Part model, mm, in its own coordinate system. Face numbers are marked on the shaded views. A direction names the side the tool comes from. Round coordinates to 2 decimals unless told otherwise and drop trailing zeros. Loops run counter-clockwise (first coordinate to the right, second up) from the corner with the lowest first, then second, coordinate; pieces in that order, holes last. Notation, with made-up numbers: M 21,89 L 72,89 A21 cw 72,96 Z; hole C 14.25,-20.5 d7. An arc over 180 degrees is marked long. Put each result on its own line as item: value. Start each with the question number.
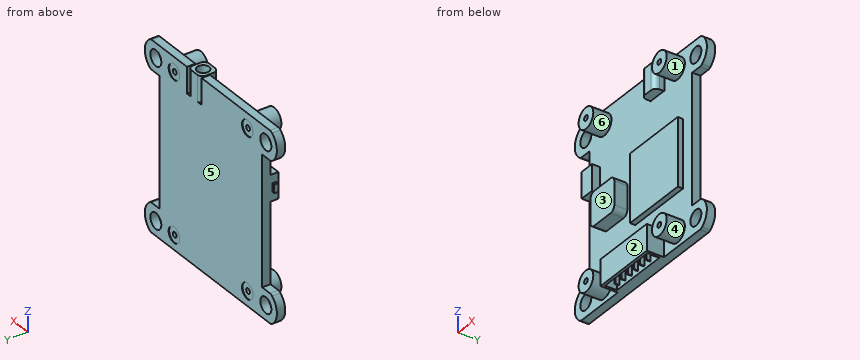
```python
from build123d import *

# Parameters (mm, degrees)
SKETCH1_R            = 1.5
SKETCH1_R_2          = 0.5
BOSS_EXTRUDE1_DEPTH  = 1.6
SKETCH2_R            = 2
SKETCH2_R_2          = 0.5
BOSS_EXTRUDE2_DEPTH  = 3.5
SKETCH3_R            = 1.5
SKETCH3_R_2          = 0.5
CUT_EXTRUDE1_DEPTH   = 0.1
SKETCH4_W            = 2.814940843
SKETCH4_H            = 5
BOSS_EXTRUDE3_DEPTH  = 1.5
SKETCH5_W            = 1.6
SKETCH5_H            = 0.8
BOSS_EXTRUDE4_DEPTH  = 0.5
BOSS_EXTRUDE5_DEPTH  = 2.5
SKETCH7_W            = 13
SKETCH7_H            = 13
BOSS_EXTRUDE6_DEPTH  = 1
SKETCH8_W            = 4
SKETCH8_H            = 1.6
CUT_EXTRUDE2_DEPTH   = 5
BOSS_EXTRUDE8_DEPTH  = 5
SKETCH10_R           = 1.15
CUT_EXTRUDE3_DEPTH   = 4
SKETCH11_W           = 12.6
SKETCH11_H           = 3.3
BOSS_EXTRUDE9_DEPTH  = 5
SKETCH12_W           = 11.6
SKETCH12_H           = 2.3
CUT_EXTRUDE4_DEPTH   = 4
SKETCH13_W           = 0.181198264
SKETCH13_H           = 0.795431403
BOSS_EXTRUDE10_DEPTH = 3.5


with BuildPart() as part:
    # Sketch1 → Boss-Extrude1 (new body)
    with BuildSketch(Plane(origin=(0, 0, 0), x_dir=(1, 0, 0), z_dir=(0, 1, 0))):
        with BuildLine():
            ThreePointArc((16.1, -18), (16.416227766, -17.948683298), (16.7, -17.8))
            ThreePointArc((16.7, -17.8), (18, -15.2), (16.7, -12.6))
            ThreePointArc((16.7, -12.6), (16.416227766, -12.451316702), (16.1, -12.4))
            Line((16.1, -12.4), (14, -12.4))
            Line((14, -12.4), (14, 12.4))
            Line((14, 12.4), (16.1, 12.4))
            ThreePointArc((16.1, 12.4), (16.416227766, 12.451316702), (16.7, 12.6))
            ThreePointArc((16.7, 12.6), (18, 15.2), (16.7, 17.8))
            ThreePointArc((16.7, 17.8), (16.416227766, 17.948683298), (16.1, 18))
            Line((16.1, 18), (-16.1, 18))
            ThreePointArc((-16.1, 18), (-16.416227766, 17.948683298), (-16.7, 17.8))
            ThreePointArc((-16.7, 17.8), (-18, 15.2), (-16.7, 12.6))
            ThreePointArc((-16.7, 12.6), (-16.416227766, 12.451316702), (-16.1, 12.4))
            Line((-16.1, 12.4), (-14, 12.4))
            Line((-14, 12.4), (-14, -12.4))
            Line((-14, -12.4), (-16.1, -12.4))
            ThreePointArc((-16.1, -12.4), (-16.416227766, -12.451316702), (-16.7, -12.6))
            ThreePointArc((-16.7, -12.6), (-18, -15.2), (-16.7, -17.8))
            ThreePointArc((-16.7, -17.8), (-16.416227766, -17.948683298), (-16.1, -18))
            Line((-16.1, -18), (16.1, -18))
        make_face()
        with Locations(Location((-15, 15.2, 0), (0, 0, 270))):
            Circle(SKETCH1_R, mode=Mode.SUBTRACT)
        with Locations(Location((15, 15.2, 0), (0, 0, 270))):
            Circle(SKETCH1_R, mode=Mode.SUBTRACT)
        with Locations(Location((-15, -15.2, 0), (0, 0, 270))):
            Circle(SKETCH1_R, mode=Mode.SUBTRACT)
        with Locations(Location((15, -15.2, 0), (0, 0, 270))):
            Circle(SKETCH1_R, mode=Mode.SUBTRACT)
        with Locations(Location((-10, -15.2, 0), (0, 0, 270))):
            Circle(SKETCH1_R_2, mode=Mode.SUBTRACT)
        with Locations(Location((10, -15.2, 0), (0, 0, 270))):
            Circle(SKETCH1_R_2, mode=Mode.SUBTRACT)
        with Locations(Location((-10, 15.2, 0), (0, 0, 270))):
            Circle(SKETCH1_R_2, mode=Mode.SUBTRACT)
        with Locations(Location((10, 15.2, 0), (0, 0, 270))):
            Circle(SKETCH1_R_2, mode=Mode.SUBTRACT)
    extrude(amount=-BOSS_EXTRUDE1_DEPTH)

    # Sketch2 → Boss-Extrude2 (add)
    # profile 1 of 4: a face of its own
    with BuildSketch(Plane.XZ.offset(1.6)):
        with Locations(Location((-10, 15.2, 0), (0, 0, 270))):
            Circle(SKETCH2_R)
        with Locations(Location((-10, 15.2, 0), (0, 0, 90))):
            Circle(SKETCH2_R_2, mode=Mode.SUBTRACT)
    # profile 2 of 4: a face of its own
    with BuildSketch(Plane.XZ.offset(1.6)):
        with Locations(Location((10, 15.2, 0), (0, 0, 90))):
            Circle(SKETCH2_R)
        with Locations(Location((10, 15.2, 0), (0, 0, 90))):
            Circle(SKETCH2_R_2, mode=Mode.SUBTRACT)
    # profile 3 of 4: a face of its own
    with BuildSketch(Plane.XZ.offset(1.6)):
        with Locations(Location((10, -15.2, 0), (0, 0, 270))):
            Circle(SKETCH2_R)
        with Locations(Location((10, -15.2, 0), (0, 0, 90))):
            Circle(SKETCH2_R_2, mode=Mode.SUBTRACT)
    # profile 4 of 4: a face of its own
    with BuildSketch(Plane.XZ.offset(1.6)):
        with Locations(Location((-10, -15.2, 0), (0, 0, 90))):
            Circle(SKETCH2_R)
        with Locations(Location((-10, -15.2, 0), (0, 0, 90))):
            Circle(SKETCH2_R_2, mode=Mode.SUBTRACT)
    extrude(amount=BOSS_EXTRUDE2_DEPTH)

    # Sketch3 → Cut-Extrude1 (cut)
    # profile 1 of 4: a face of its own
    with BuildSketch(Plane(origin=(0, 0, 0), x_dir=(1, 0, 0), z_dir=(0, 1, 0))):
        with Locations(Location((-10, 15.2, 0), (0, 0, 270))):
            Circle(SKETCH3_R)
        with Locations(Location((-10, 15.2, 0), (0, 0, 270))):
            Circle(SKETCH3_R_2, mode=Mode.SUBTRACT)
    # profile 2 of 4: a face of its own
    with BuildSketch(Plane(origin=(0, 0, 0), x_dir=(1, 0, 0), z_dir=(0, 1, 0))):
        with Locations(Location((10, 15.2, 0), (0, 0, 90))):
            Circle(SKETCH3_R)
        with Locations(Location((10, 15.2, 0), (0, 0, 270))):
            Circle(SKETCH3_R_2, mode=Mode.SUBTRACT)
    # profile 3 of 4: a face of its own
    with BuildSketch(Plane(origin=(0, 0, 0), x_dir=(1, 0, 0), z_dir=(0, 1, 0))):
        with Locations(Location((10, -15.2, 0), (0, 0, 270))):
            Circle(SKETCH3_R)
        with Locations(Location((10, -15.2, 0), (0, 0, 270))):
            Circle(SKETCH3_R_2, mode=Mode.SUBTRACT)
    # profile 4 of 4: a face of its own
    with BuildSketch(Plane(origin=(0, 0, 0), x_dir=(1, 0, 0), z_dir=(0, 1, 0))):
        with Locations(Location((-10, -15.2, 0), (0, 0, 90))):
            Circle(SKETCH3_R)
        with Locations(Location((-10, -15.2, 0), (0, 0, 270))):
            Circle(SKETCH3_R_2, mode=Mode.SUBTRACT)
    extrude(amount=-CUT_EXTRUDE1_DEPTH, mode=Mode.SUBTRACT)

    # Sketch4 → Boss-Extrude3 (add)
    with BuildSketch(Plane.XZ.offset(1.6)):
        with Locations((-12.592529579, 5.5)):
            Rectangle(SKETCH4_W, SKETCH4_H)
    extrude(amount=BOSS_EXTRUDE3_DEPTH)

    # Sketch5 → Boss-Extrude4 (add)
    with BuildSketch(Plane.ZY.offset(14)):
        with Locations((5.5, -2.35)):
            Rectangle(SKETCH5_W, SKETCH5_H)
    extrude(amount=BOSS_EXTRUDE4_DEPTH)

    # Sketch6 → Boss-Extrude5 (add)
    with BuildSketch(Plane.XZ.offset(1.6)):
        with BuildLine():
            Line((-9.180413125, 1.55720135), (-4.680413125, 1.55720135))
            ThreePointArc((-4.680413125, 1.55720135), (-3.973306344, 1.264308131), (-3.680413125, 0.55720135))
            Line((-3.680413125, 0.55720135), (-3.680413125, -3.94279865))
            ThreePointArc((-3.680413125, -3.94279865), (-3.973306344, -4.649905431), (-4.680413125, -4.94279865))
            Line((-4.680413125, -4.94279865), (-9.180413125, -4.94279865))
            ThreePointArc((-9.180413125, -4.94279865), (-9.887519906, -4.649905431), (-10.180413125, -3.94279865))
            Line((-10.180413125, -3.94279865), (-10.180413125, 0.55720135))
            ThreePointArc((-10.180413125, 0.55720135), (-9.887519906, 1.264308131), (-9.180413125, 1.55720135))
        make_face()
    extrude(amount=BOSS_EXTRUDE5_DEPTH)

    # Sketch7 → Boss-Extrude6 (add)
    with BuildSketch(Plane.XZ.offset(1.6)):
        with Locations((4.986452967, -1.419959553)):
            Rectangle(SKETCH7_W, SKETCH7_H)
    extrude(amount=BOSS_EXTRUDE6_DEPTH)

    # Sketch8 → Cut-Extrude2 (cut)
    with BuildSketch(Plane.XY.offset(18)):
        with Locations((4.5, -0.8)):
            Rectangle(SKETCH8_W, SKETCH8_H)
    extrude(amount=-CUT_EXTRUDE2_DEPTH, mode=Mode.SUBTRACT)

    # Sketch9 → Boss-Extrude8 (add)
    with BuildSketch(Plane.XY.offset(13)):
        with BuildLine():
            Line((3.702131482, 0), (5.287124598, 0))
            ThreePointArc((5.287124598, 0), (5.994231379, -0.292893219), (6.287124598, -1))
            Line((6.287124598, -1), (6.287124598, -2.4))
            ThreePointArc((6.287124598, -2.4), (5.994231379, -3.107106781), (5.287124598, -3.4))
            Line((5.287124598, -3.4), (3.702131482, -3.4))
            ThreePointArc((3.702131482, -3.4), (2.995024701, -3.107106781), (2.702131482, -2.4))
            Line((2.702131482, -2.4), (2.702131482, -1))
            ThreePointArc((2.702131482, -1), (2.995024701, -0.292893219), (3.702131482, 0))
        make_face()
    extrude(amount=BOSS_EXTRUDE8_DEPTH)

    # Sketch10 → Cut-Extrude3 (cut)
    with BuildSketch(Plane.XY.offset(18)):
        with Locations((4.49462804, -1.7)):
            Circle(SKETCH10_R)
    extrude(amount=-CUT_EXTRUDE3_DEPTH, mode=Mode.SUBTRACT)

    # Sketch11 → Boss-Extrude9 (add)
    with BuildSketch(Plane(origin=(0, 0, -18), x_dir=(-1, 0, 0), z_dir=(0, 0, -1))):
        with Locations((0, -3.25)):
            Rectangle(SKETCH11_W, SKETCH11_H)
    extrude(amount=-BOSS_EXTRUDE9_DEPTH)

    # Sketch12 → Cut-Extrude4 (cut)
    with BuildSketch(Plane(origin=(0, 0, -18), x_dir=(-1, 0, 0), z_dir=(0, 0, -1))):
        with Locations((0, -3.25)):
            Rectangle(SKETCH12_W, SKETCH12_H)
    extrude(amount=-CUT_EXTRUDE4_DEPTH, mode=Mode.SUBTRACT)

    # Sketch13 → Boss-Extrude10 (add)
    with BuildSketch(Plane(origin=(0, 0, -14), x_dir=(-1, 0, 0), z_dir=(0, 0, -1))):
        with Locations((-5.139752883, -2.609229229)):
            Rectangle(SKETCH13_W, SKETCH13_H)
        with Locations((-3.439752883, -2.609229229)):
            Rectangle(SKETCH13_W, SKETCH13_H)
        with Locations((-1.739752883, -2.609229229)):
            Rectangle(SKETCH13_W, SKETCH13_H)
        with Locations((-0.039752883, -2.609229229)):
            Rectangle(SKETCH13_W, SKETCH13_H)
        with Locations((1.660247117, -2.609229229)):
            Rectangle(SKETCH13_W, SKETCH13_H)
        with Locations((3.360247117, -2.609229229)):
            Rectangle(SKETCH13_W, SKETCH13_H)
        with Locations((5.060247117, -2.609229229)):
            Rectangle(SKETCH13_W, SKETCH13_H)
    extrude(amount=BOSS_EXTRUDE10_DEPTH)


solid = part.part
```
1. Cut at A-A, the plane x = 15. Give the cut face in (y, z), and give its area (3 significant figures).
2. Wall check: L1, parallel to X at y = -0.05, z = -15.2; L2, parallel to X at y = -4.1, z = -15.2; L3, parallel to X at y = -1.15, z = -15.2. Give the ranges that are in metal, low to high.
3. Cut at B-B, the plane x = 10. Give the number of separate pieces and of enclosed holes in the cut face, and give its area (3 significant figures).
4. Drop flat-ended pins along their axis: pin 1 (12 mm diameter, centred on x = -5, z = 3.5, fed in from -Y); pin 2 (1 mm diameter, centred on y = -3.5, z = -1.5, fed in from -X); pin 3 (1.2 mm diameter, centred on x = 0.5, z = -16, fed in from -Y); pin 4 (1 mm diameter, centred on y = -4, z = 12, fed in from +X). Give the stop position or say it passes through.
5. Which spindle directions (+Z, -Z, +X, -X, +Y, -Y) get a long thin tool onto all of the face, cutting with end or side? Do the marked faces 1, 2 and 3. Say none if no direction does.
6. Mould opens along X. For the marked faces 4, 5 and 6 say: released by +X, released by -X, zero draft, split by the parting line, or undercut.
7. Cut at C-C, the plane z = -6.5. Give the cut face in (x, y), and give its area (3 significant figures).
8. Cut at D-D, the plane x = 1. Give the cut face in (y, z).
Results list:
1. outline: M -1.6,-18 L 0,-18 L 0,-16.7 L -1.6,-16.7 Z; M -1.6,-13.7 L 0,-13.7 L 0,-12.4 L -1.6,-12.4 Z; M -1.6,12.4 L 0,12.4 L 0,13.7 L -1.6,13.7 Z; M -1.6,16.7 L 0,16.7 L 0,18 L -1.6,18 Z
1. area: 8.32 mm^2
2. L1: x = -18 to -16.5, -13.5 to -11.5, -8.5 to 8.5, 11.5 to 13.5, 16.5 to 18
2. L2: x = -12 to -10.5, -9.5 to -8, -6.3 to -5.8, 5.8 to 6.3, 8 to 9.5, 10.5 to 12
2. L3: x = -18 to -16.5, -13.5 to -10.5, -9.5 to 9.5, 10.5 to 13.5, 16.5 to 18
3. separate pieces: 3
3. enclosed holes: 0
3. area: 88.0 mm^2
4. pin 1: stops at y = -4.1
4. pin 2: stops at x = -10.18
4. pin 3: stops at y = -4.9
4. pin 4: passes through
5. face 1: -Y
5. face 2: +Z, -Z, -Y
5. face 3: +X, -X, -Y
6. face 4: undercut
6. face 5: zero draft
6. face 6: undercut
7. outline: M -14,-1.6 L -1.51,-1.6 L -1.51,-2.6 L 11.49,-2.6 L 11.49,-1.6 L 14,-1.6 L 14,0 L -14,0 Z
7. area: 57.8 mm^2
8. outline: M -4.9,-18 L -4.4,-18 L -4.4,-14 L -2.1,-14 L -2.1,-18 L 0,-18 L 0,18 L -1.6,18 L -1.6,5.08 L -2.6,5.08 L -2.6,-7.92 L -1.6,-7.92 L -1.6,-13 L -4.9,-13 Z
